Read the model definition and answer for the solid it produces. Units are mm, in the model's axes. Face numbers are marked on the shaded views. Give positions to 0.01 mm unless a question says otherwise; leave off trailing zeros. Order: outer loops, then holes, each group sorted by start corner. A loop starts at its lowest first (then second) coordinate and runs counter-clockwise, first axis right, second up.
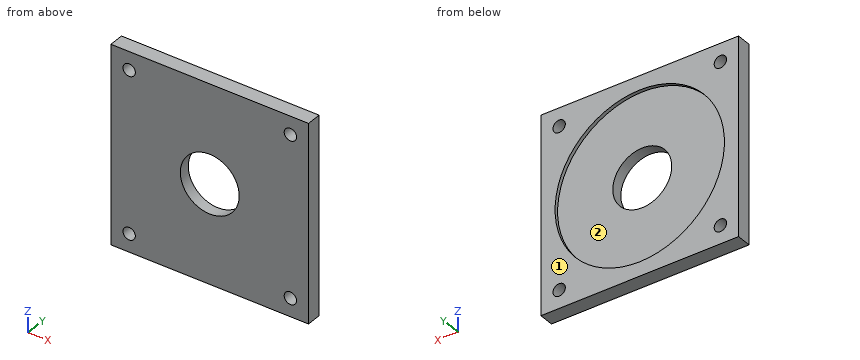
```python
from build123d import *

# Parameters (mm, degrees)
SKETCH1_W           = 85.2
SKETCH1_H           = 85.2
BOSS_EXTRUDE1_DEPTH = 6.35
CUT_EXTRUDE1_REACH  = 62.579
SKETCH2_R           = 36.49
BOSS_EXTRUDE2_START = -4.83
SKETCH5_R           = 36.49
SKETCH5_R_2         = 12.7
BOSS_EXTRUDE2_DEPTH = 4.83
CUT_EXTRUDE2_REACH  = 62.579
SKETCH6_R           = 2.665


with BuildPart() as part:
    # Sketch1 → Boss-Extrude1 (new body)
    with BuildSketch(Plane(origin=(0, 0, 0), x_dir=(1, 0, 0), z_dir=(0, 1, 0))):
        Rectangle(SKETCH1_W, SKETCH1_H)
    extrude(amount=BOSS_EXTRUDE1_DEPTH)

    # Sketch2 → Cut-Extrude1 (cut, up to next)
    with BuildSketch(Plane(origin=(0, 6.35, 0), x_dir=(1, 0, 0), z_dir=(0, 1, 0)), mode=Mode.PRIVATE) as cut_extrude1_sk1:
        with Locations(Location((0, 0, 0), (0, 0, 270))):
            Circle(SKETCH2_R)
    cut_extrude1_tool1 = extrude(cut_extrude1_sk1.sketch, amount=-CUT_EXTRUDE1_REACH, mode=Mode.PRIVATE) & part.part
    add(cut_extrude1_tool1.solids().sort_by_distance((0, 6.35, 0))[0], mode=Mode.SUBTRACT)

    # Sketch5 → Boss-Extrude2 (add)
    with BuildSketch(Plane.XZ.offset(BOSS_EXTRUDE2_START)):
        with Locations(Location((0, 0, 0), (0, 0, 90))):
            Circle(SKETCH5_R)
        with Locations(Location((0, 0, 0), (0, 0, 270))):
            Circle(SKETCH5_R_2, mode=Mode.SUBTRACT)
    extrude(amount=BOSS_EXTRUDE2_DEPTH)

    # Sketch6 → Cut-Extrude2 (cut, up to next)
    with BuildSketch(Plane.XZ, mode=Mode.PRIVATE) as cut_extrude2_sk1:
        with Locations(Location((-34.75, -34.75, 0), (0, 0, 270))):
            Circle(SKETCH6_R)
    cut_extrude2_tool1 = extrude(cut_extrude2_sk1.sketch, amount=-CUT_EXTRUDE2_REACH, mode=Mode.PRIVATE) & part.part
    # Sketch6 → Cut-Extrude2 (cut, up to next)
    with BuildSketch(Plane.XZ, mode=Mode.PRIVATE) as cut_extrude2_sk2:
        with Locations(Location((-34.75, 34.75, 0), (0, 0, 270))):
            Circle(SKETCH6_R)
    cut_extrude2_tool2 = extrude(cut_extrude2_sk2.sketch, amount=-CUT_EXTRUDE2_REACH, mode=Mode.PRIVATE) & part.part
    # Sketch6 → Cut-Extrude2 (cut, up to next)
    with BuildSketch(Plane.XZ, mode=Mode.PRIVATE) as cut_extrude2_sk3:
        with Locations(Location((34.75, 34.75, 0), (0, 0, 270))):
            Circle(SKETCH6_R)
    cut_extrude2_tool3 = extrude(cut_extrude2_sk3.sketch, amount=-CUT_EXTRUDE2_REACH, mode=Mode.PRIVATE) & part.part
    # Sketch6 → Cut-Extrude2 (cut, up to next)
    with BuildSketch(Plane.XZ, mode=Mode.PRIVATE) as cut_extrude2_sk4:
        with Locations(Location((34.75, -34.75, 0), (0, 0, 270))):
            Circle(SKETCH6_R)
    cut_extrude2_tool4 = extrude(cut_extrude2_sk4.sketch, amount=-CUT_EXTRUDE2_REACH, mode=Mode.PRIVATE) & part.part
    add(cut_extrude2_tool1.solids().sort_by_distance((-34.75, 0, -34.75))[0], mode=Mode.SUBTRACT)
    add(cut_extrude2_tool2.solids().sort_by_distance((-34.75, 0, 34.75))[0], mode=Mode.SUBTRACT)
    add(cut_extrude2_tool3.solids().sort_by_distance((34.75, 0, 34.75))[0], mode=Mode.SUBTRACT)
    add(cut_extrude2_tool4.solids().sort_by_distance((34.75, 0, -34.75))[0], mode=Mode.SUBTRACT)


solid = part.part
```
1) The part is cut by section C-C on x = 5.5. Determine the outline of the cut face in (y, z), and give its area (3 significant figures).
Final values:
outline: (0, -42.6) - (6.35, -42.6) - (6.35, -36.07) - (4.83, -36.07) - (4.83, -11.45) - (0, -11.45) - close; (0, 11.45) - (4.83, 11.45) - (4.83, 36.07) - (6.35, 36.07) - (6.35, 42.6) - (0, 42.6) - close
area: 321 mm2
2) The part is cut by section B-B on z = 0. Determine the outline of the cut face in (x, y), and give its area (3 significant figures).
Final values:
outline: (-42.6, 0) - (-12.7, 0) - (-12.7, 4.83) - (-36.49, 4.83) - (-36.49, 6.35) - (-42.6, 6.35) - close; (12.7, 0) - (42.6, 0) - (42.6, 6.35) - (36.49, 6.35) - (36.49, 4.83) - (12.7, 4.83) - close
area: 307 mm2
3) For a pull along Z with two mould halves and no side action, classify the marked faces 1 and 2 as released by +Z, released by -Z, zero draft, split by the parting line, or undercut.
Final values:
face 1: zero draft
face 2: undercut
4) The part is cut by section D-D on x = 34.75. Determine the outline of the cut face in (y, z) (3 decimals).
Final values:
outline: (0, -42.6) - (6.35, -42.6) - (6.35, -37.415) - (0, -37.415) - close; (0, -32.085) - (6.35, -32.085) - (6.35, -11.134) - (4.83, -11.134) - (4.83, 11.134) - (6.35, 11.134) - (6.35, 32.085) - (0, 32.085) - close; (0, 37.415) - (6.35, 37.415) - (6.35, 42.6) - (0, 42.6) - close
5) The part is cut by section A-A on y = 3.5. Determine the outline of the cut face in (x, z) (3 decimals).
Final values:
outline: (-42.6, -42.6) - (42.6, -42.6) - (42.6, 42.6) - (-42.6, 42.6) - close; hole circle Ø5.33 at (-34.75, -34.75); hole circle Ø5.33 at (-34.75, 34.75); hole circle Ø25.4 at (0, 0); hole circle Ø5.33 at (34.75, -34.75); hole circle Ø5.33 at (34.75, 34.75)
6) Given pin 1 (3 mm diameter, centred on x = -34.75, z = 34.75, fed in from -Y); pin 2 (3 mm diameter, centred on x = -9.5, z = -10, fed in from +Y), each flat-ended and moving along its own axis, determine where each tip first touches the part or whether it passes through.
Final values:
pin 1: passes through
pin 2: stops at y = 4.83
7) Consider L1, parallel to X at y = 4.25, z = -34.75 (3 decimals); L2, parallel to X at y = 1.35, z = 0; L3, parallel to X at y = 1.5, z = -34. Determine where each line is inside the solid, lowest interval first.
Final values:
L1: x = -42.6 to -37.415, -32.085 to 32.085, 37.415 to 42.6
L2: x = -42.6 to -12.7, 12.7 to 42.6
L3: x = -42.6 to -37.31, -32.19 to 32.19, 37.31 to 42.6
